```python
from build123d import *

# Parameters (mm, degrees)
SKETCH1_W           = 122
SKETCH1_H           = 52
SKETCH1_R           = 2.9
SKETCH1_R_2         = 6
SKETCH1_R_3         = 5.5
SKETCH1_W_2         = 62.4
SKETCH1_H_2         = 50
SKETCH1_R_4         = 1.6
BOSS_EXTRUDE1_DEPTH = 4
SKETCH1_3_W         = 4
SKETCH1_3_H         = 52
BOSS_EXTRUDE2_DEPTH = 50
SKETCH3_R           = 1.25
CUT_EXTRUDE1_DEPTH  = 104.879216611
FILLET2_R           = 5
FILLET3_R           = 5
FILLET4_R           = 5
FILLET5_R           = 5
FILLET6_R           = 5


# Some blends are built 0.0001 mm under size
with BuildPart() as part:
    # Sketch1 → Boss-Extrude1 (new body)
    with BuildSketch(Plane.XY):
        with Locations((3.490084273, -6.001542194)):
            Rectangle(SKETCH1_W, SKETCH1_H)
        with Locations((-53.509915727, -27.501542194)):
            Circle(SKETCH1_R, mode=Mode.SUBTRACT)
        with Locations((-44.509915727, -27.501542194)):
            Circle(SKETCH1_R, mode=Mode.SUBTRACT)
        with Locations((-49.009915727, -21.001542194)):
            Circle(SKETCH1_R, mode=Mode.SUBTRACT)
        with Locations((-32.009915727, -21.001542194)):
            Circle(SKETCH1_R_2, mode=Mode.SUBTRACT)
        with Locations((-49.009915727, -6.001542194)):
            Circle(SKETCH1_R_3, mode=Mode.SUBTRACT)
        with Locations((-32.009915727, -6.001542194)):
            Circle(SKETCH1_R_3, mode=Mode.SUBTRACT)
        with Locations((-49.009915727, 8.998457806)):
            Circle(SKETCH1_R_3, mode=Mode.SUBTRACT)
        with Locations((-32.009915727, 8.998457806)):
            Circle(SKETCH1_R_3, mode=Mode.SUBTRACT)
        with Locations((26.390084273, -6.001542194)):
            Rectangle(SKETCH1_W_2, SKETCH1_H_2, mode=Mode.SUBTRACT)
        with Locations((-15.089915727, 15.448457806)):
            Circle(SKETCH1_R_4, mode=Mode.SUBTRACT)
        with Locations((-15.089915727, -28.451542194)):
            Circle(SKETCH1_R_4, mode=Mode.SUBTRACT)
        with Locations((61.010084273, 15.448457806)):
            Circle(SKETCH1_R_4, mode=Mode.SUBTRACT)
        with Locations((61.010084273, -28.451542194)):
            Circle(SKETCH1_R_4, mode=Mode.SUBTRACT)
    extrude(amount=-BOSS_EXTRUDE1_DEPTH)

    # Sketch1<3> → Boss-Extrude2 (add)
    with BuildSketch(Plane.XY):
        Polygon((68.490084273, 23.998457806), (-61.509915727, 23.998457806), (-61.509915727, 19.998457806), (-57.509915727, 19.998457806), (64.490084273, 19.998457806), (68.490084273, 19.998457806), align=None)
        with Locations((-59.509915727, -6.001542194)):
            Rectangle(SKETCH1_3_W, SKETCH1_3_H)
        with Locations((66.490084273, -6.001542194)):
            Rectangle(SKETCH1_3_W, SKETCH1_3_H)
        Polygon((-57.509915727, -32.001542194), (-61.509915727, -32.001542194), (-61.509915727, -36.001542194), (68.490084273, -36.001542194), (68.490084273, -32.001542194), (64.490084273, -32.001542194), align=None)
    extrude(amount=-BOSS_EXTRUDE2_DEPTH)

    # Sketch3 → Cut-Extrude1 (cut, through all)
    with BuildSketch(Plane(origin=(0, 23.998457806, 0), x_dir=(1, 0, 0), z_dir=(0, 1, 0))):
        with Locations(Location((-51.509915727, 47, 0), (0, 0, 270))):
            Circle(SKETCH3_R)
        with Locations(Location((58.490084273, 47, 0), (0, 0, 270))):
            Circle(SKETCH3_R)
    extrude(amount=-CUT_EXTRUDE1_DEPTH, mode=Mode.SUBTRACT)

    # Fillet2
    fillet2_edges = [part.edges().sort_by_distance(p)[0] for p in [
        (-61.509915727, -6.001542194, 0),
    ]]
    fillet(fillet2_edges, radius=FILLET2_R)

    # Fillet3
    fillet3_edges = [part.edges().sort_by_distance(p)[0] for p in [
        (68.490084273, -6.001542194, 0),
    ]]
    fillet(fillet3_edges, radius=FILLET3_R)

    # Fillet4
    fillet4_edges = [part.edges().sort_by_distance(p)[0] for p in [
        (3.490084273, 23.998457806, 0),
        (-60.045449633, 23.998457806, -1.464466094),
        (67.025618179, 23.998457806, -1.464466094),
        (-61.509915727, 23.998457806, -27.5),
        (68.490084273, 23.998457806, -27.5),
    ]]
    fillet(fillet4_edges, radius=FILLET4_R - 0.0001)  # a hair under: the kernel refuses the full size

    # Fillet5
    fillet5_edges = [part.edges().sort_by_distance(p)[0] for p in [
        (-60.045449633, -36.001542194, -1.464466094),
        (3.490084273, -36.001542194, 0),
        (67.025618179, -36.001542194, -1.464466094),
        (68.490084273, -36.001542194, -27.5),
        (-61.509915727, -36.001542194, -27.5),
    ]]
    fillet(fillet5_edges, radius=FILLET5_R - 0.0001)  # a hair under: the kernel refuses the full size

    # Fillet6
    # the kernel refuses this fillet: 5 mm, written as the material it takes off along each edge
    with BuildSketch(Plane(origin=(-56.510015727, 18.998557806, -50), x_dir=(-1, 0, 0), z_dir=(0, -1, 0))) as fillet6_piece_1:
        with BuildLine():
            CenterArc((0, -4.9999), FILLET6_R, 0, 90)
            Line((5, -4.9999), (5.1, -4.9999))
            ThreePointArc((5.1, -4.9999), (5.0999, -2.49995), (5.0999, 0))
            Line((5.0999, 0), (4.9999, 0.1))
            ThreePointArc((4.9999, 0.1), (2.49995, 0.1), (0, 0.1001))
            Line((0, 0.1001), (0, 0.0001))
        make_face()
    revolve(axis=Axis((-56.510015727, 18.998557806, -50), (0, 0, -1)), revolution_arc=90, mode=Mode.SUBTRACT)
    with BuildSketch(Plane(origin=(-61.509915727, 18.998557806, -50), x_dir=(-2.0000400003242763e-05, 0, 0.9999999997999919), z_dir=(0, -1, 0)), Plane(origin=(68.490084273, -31.001642194, -50), x_dir=(2.0000400004663874e-05, 0, 0.9999999997999919), z_dir=(0, 1, 0))) as fillet6_piece_2:
        with BuildLine():
            CenterArc((4.999799999, -4.999999999), FILLET6_R, 89.998854061, 90)
            Line((-0.0002, -4.999899997), (-0.1002, -4.999897997))
            ThreePointArc((-0.1002, -4.999897997), (-0.10005, -2.499947999), (-0.1, 2e-06))
            Line((-0.1, 2e-06), (2e-06, 0.1))
            ThreePointArc((2e-06, 0.1), (2.499952, 0.09995), (4.999902001, 0.1))
            Line((4.999902001, 0.1), (4.999900001, 0))
        make_face()
    extrude(amount=50.0002, mode=Mode.SUBTRACT)
    with BuildSketch(Plane(origin=(-56.510015727, -31.001642194, -50), x_dir=(0, -1, 0), z_dir=(1, 0, 0))) as fillet6_piece_3:
        with BuildLine():
            CenterArc((0, -4.9999), FILLET6_R, 0, 90)
            Line((5, -4.9999), (5.1, -4.9999))
            ThreePointArc((5.1, -4.9999), (5.0999, -2.49995), (5.0999, 0))
            Line((5.0999, 0), (4.9999, 0.1))
            ThreePointArc((4.9999, 0.1), (2.49995, 0.1), (0, 0.1001))
            Line((0, 0.1001), (0, 0.0001))
        make_face()
    revolve(axis=Axis((-56.510015727, -31.001642194, -50), (0, 0, -1)), revolution_arc=90, mode=Mode.SUBTRACT)
    with BuildSketch(Plane(origin=(-56.510015727, -36.001542194, -50), x_dir=(0, -2.0000400004663874e-05, 0.9999999997999919), z_dir=(1, 0, 0)), Plane(origin=(63.490184273, 23.998457806, -50), x_dir=(0, 2.000040000395332e-05, 0.9999999997999919), z_dir=(-1, 0, 0))) as fillet6_piece_4:
        with BuildLine():
            CenterArc((4.999799999, -4.999999999), FILLET6_R, 89.998854061, 90)
            Line((-0.0002, -4.999899997), (-0.1002, -4.999897997))
            ThreePointArc((-0.1002, -4.999897997), (-0.10005, -2.499947999), (-0.1, 2e-06))
            Line((-0.1, 2e-06), (2e-06, 0.1))
            ThreePointArc((2e-06, 0.1), (2.499952, 0.09995), (4.999902001, 0.1))
            Line((4.999902001, 0.1), (4.999900001, 0))
        make_face()
    extrude(amount=120.0002, mode=Mode.SUBTRACT)
    with BuildSketch(Plane(origin=(63.490184273, -31.001642194, -50), x_dir=(0, -1, 0), z_dir=(-1, 0, 0))) as fillet6_piece_5:
        with BuildLine():
            CenterArc((0, 4.9999), FILLET6_R, 270, 90)
            Line((0, -0.0001), (0, -0.1001))
            ThreePointArc((0, -0.1001), (2.49995, -0.1), (4.9999, -0.1))
            Line((4.9999, -0.1), (5.0999, 0))
            ThreePointArc((5.0999, 0), (5.0999, 2.49995), (5.1, 4.9999))
            Line((5.1, 4.9999), (5, 4.9999))
        make_face()
    revolve(axis=Axis((63.490184273, -31.001642194, -50), (0, 0, 1)), revolution_arc=90, mode=Mode.SUBTRACT)
    with BuildSketch(Plane(origin=(63.490184273, 18.998557806, -50), x_dir=(1, 0, 0), z_dir=(0, -1, 0))) as fillet6_piece_6:
        with BuildLine():
            CenterArc((0, 4.9999), FILLET6_R, 270, 90)
            Line((0, -0.0001), (0, -0.1001))
            ThreePointArc((0, -0.1001), (2.49995, -0.1), (4.9999, -0.1))
            Line((4.9999, -0.1), (5.0999, 0))
            ThreePointArc((5.0999, 0), (5.0999, 2.49995), (5.1, 4.9999))
            Line((5.1, 4.9999), (5, 4.9999))
        make_face()
    revolve(axis=Axis((63.490184273, 18.998557806, -50), (0, 0, 1)), revolution_arc=90, mode=Mode.SUBTRACT)


solid = part.part
```
Source: CAD feature listing. Evaluate the final solid. Frame: model axes, mm. A direction names the side the tool comes from. Give positions to 0.01 mm unless a question says otherwise; leave off trailing zeros. Loops run counter-clockwise (first coordinate to the right, second up) from the corner with the lowest first, then second, coordinate; pieces in that order, holes last. Notation, with made-up numbers: (17.25, 26.5) -> (53.25, 26.5) arc R17 cw to (53.25, 42.5) -> close; hole circle Ø11 at (60, 13). An arc over 180 degrees is marked (long way). Use a Markdown table: item, result. Add a question column.
(1) First-contact query: pin 1 Ø1 at (x, y) = (-18.5, -18.5) entering from +Z; pin 2 Ø1 at (x, y) = (25, 18) entering from -Z; pin 3 Ø1.2 at (y, z) = (1, -2.5) entering from +X (3 decimals); pin 4 Ø3 at (x, z) = (-51.51, -47) entering from -Y. Flat tips, straight axial feed; report the tip coordinate or a pass-through.
(2) Section query A-A (y = 2). Output: boundary loops of the cut face in (x, z).
(3) Ray query, line 1 (Y direction, x = -26.5, z = -41); line 2 (X direction, y = -6, z = -29); line 3 (X direction, y = 22.3, z = -47). Return the intervals inside material, ascending.
(4) Section query B-B (z = -26.5). Output: boundary loops of the cut face in (x, y), then the cut area to 3 significant figures.
(5) Pull-direction query (Y, two-part tool) for faces 4 (the face through (3, 23, -2)), 5 (the face through (68.49, -6, -25)), 6 (the face through (3, -35, -48)), 7 (the face through (64.49, -6, -27)); classes: +Y half, -Y half, draft (parallel to the pull), parting line (faces both ways), or undercut.
(6) Access query for faces 1 (the face through (3, 19.998, -27)), 2 (the face through (-60.4, -5.65, -48.14)), 3 (the face through (26, -31.002, -2)). Directions: +Z, -Z, +X, -X, +Y, -Y. A direction counts if a zero-diameter tool reaches every point of the face in a straight line with its end or side. Return the directions, or none.
(7) Section query D-D (z = -47). Output: boundary loops of the cut face in (x, y).
Checked values:
| question | item | result |
|---|---|---|
| 1 | pin 1 | z = 0 |
| 1 | pin 2 | through |
| 1 | pin 3 | x = 68.115 |
| 1 | pin 4 | y = -35.98 |
| 2 | outline | (-61.51, -45.03) arc R5 ccw to (-57.51, -49.9) -> (-57.51, -4) -> (-4.81, -4) -> (-4.81, 0) -> (-56.51, 0) arc R5 ccw to (-61.51, -5) -> close; (57.59, -4) -> (64.49, -4) -> (64.49, -49.9) arc R5 ccw to (68.49, -45.03) -> (68.49, -5) arc R5 ccw to (63.49, 0) -> (57.59, 0) -> close |
| 3 | line 1 | -36 to -32, 20 to 24 |
| 3 | line 2 | -61.51 to -57.51, 64.49 to 68.49 |
| 3 | line 3 | -59.69 to -52.76, -50.26 to 57.24, 59.74 to 66.67 |
| 4 | outline | (-61.51, -31) arc R5 ccw to (-56.51, -36) -> (63.49, -36) arc R5 ccw to (68.49, -31) -> (68.49, 19) arc R5 ccw to (63.49, 24) -> (-56.51, 24) arc R5 ccw to (-61.51, 19) -> close; hole (-57.51, -32) -> (64.49, -32) -> (64.49, 20) -> (-57.51, 20) -> close |
| 4 | area | 1,430 mm^2 |
| 5 | face 4 | +Y half |
| 5 | face 5 | draft |
| 5 | face 6 | -Y half |
| 5 | face 7 | undercut |
| 6 | face 1 | -Z |
| 6 | face 2 | -Z, -X, +Y, -Y |
| 6 | face 3 | +Z, -Z |
| 7 | outline | (-61.09, -31) arc R4.58 ccw to (-56.51, -35.58) -> (-52.76, -35.58) -> (-52.76, -32) -> (-57.51, -32) -> (-57.51, 20) -> (-52.76, 20) -> (-52.76, 23.58) -> (-56.51, 23.58) arc R4.58 ccw to (-61.09, 19) -> close; (-50.26, -35.58) -> (57.24, -35.58) -> (57.24, -32) -> (-50.26, -32) -> close; (-50.26, 20) -> (57.24, 20) -> (57.24, 23.58) -> (-50.26, 23.58) -> close; (59.74, -35.58) -> (63.49, -35.58) arc R4.58 ccw to (68.07, -31) -> (68.07, 19) arc R4.58 ccw to (63.49, 23.58) -> (59.74, 23.58) -> (59.74, 20) -> (64.49, 20) -> (64.49, -32) -> (59.74, -32) -> close |
